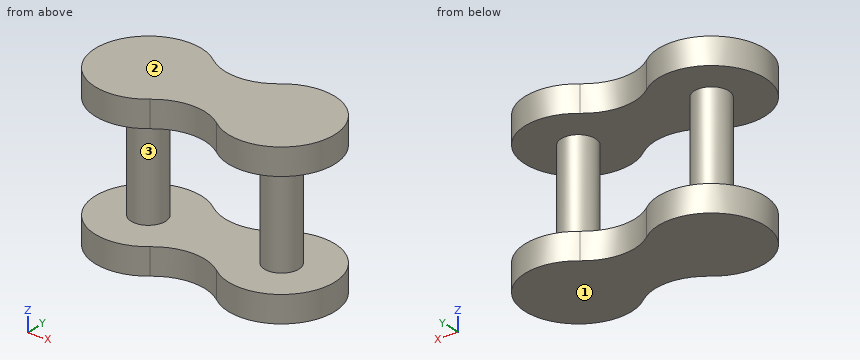
from build123d import *

# Parameters (mm, degrees)
SKETCH1_R             = 0.8255
BOSS_EXTRUDE1_DEPTH   = 2.54
BOSS_EXTRUDE1_2_DEPTH = 2.54
BOSS_EXTRUDE2_DEPTH   = 1.27


with BuildPart() as part:
    # Sketch1 → Boss-Extrude1 (new, symmetric)
    with BuildSketch(Plane.XY):
        with Locations((3.175, 0)):
            Circle(SKETCH1_R)
    extrude(amount=BOSS_EXTRUDE1_DEPTH, both=True)



with BuildPart() as body_2:
    # Sketch1 → Boss-Extrude1 2 (new, symmetric)
    with BuildSketch(Plane.XY):
        with Locations((-3.175, 0)):
            Circle(SKETCH1_R)
    extrude(amount=BOSS_EXTRUDE1_2_DEPTH, both=True)


with BuildPart() as part_1:
    add(part.part)

    add(body_2.part)  # Boss-Extrude2 merges body 2
    # Sketch2 → Boss-Extrude2 (add)
    with BuildSketch(Plane.XY.offset(2.54)):
        with BuildLine():
            ThreePointArc((1.5875, -1.982786864), (5.715, 0), (1.5875, 1.982786864))
            ThreePointArc((1.5875, 1.982786864), (0, 1.425573729), (-1.5875, 1.982786864))
            ThreePointArc((-1.5875, 1.982786864), (-5.715, 0), (-1.5875, -1.982786864))
            ThreePointArc((-1.5875, -1.982786864), (0, -1.425573729), (1.5875, -1.982786864))
        make_face()
    boss_extrude2 = extrude(amount=BOSS_EXTRUDE2_DEPTH)

    # Mirror1: Boss-Extrude2 across plane
    add(boss_extrude2.mirror(Plane.XY))


solid = part_1.part
Read the model definition and answer for the solid it produces. Units are mm, in the model's axes. Face numbers are marked on the shaded views. Coordinates: 2 decimals unless noted, no trailing zeros. Loops run counter-clockwise (first coordinate to the right, second up) from the corner with the lowest first, then second, coordinate; pieces in that order, holes last.
Q1. Consider probe 1 along Z at (x, y) = (-2.75, -1.7); probe 2 along X at (y, z) = (-0.7, -1.5); probe 3 along X at (y, z) = (0.45, 3). Determine where each line is inside the solid, lowest interval first.
Q2. The part is cut by section D-D on z = -0.25. Write down the section's boundary in (x, y) (1 decimal), and give its area (3 significant figures).
Q3. The part is cut by section A-A on y = 0. Write down the section's boundary in (x, z) (1 decimal).
Q4. The part is cut by section C-C on y = -2.2. Write down the section's boundary in (x, z), and give its area (3 significant figures).
Q5. The mould has two halves that part along Z. Classify the marked faces 1, 2 and 3: +Z half, -Z half, draft (parallel to the pull), parting line (faces both ways), or undercut.
Q6. The part is cut by section B-B on x = 1.75. Write down the section's boundary in (y, z).
Results below:
1. probe 1: z = -3.81 to -2.54, 2.54 to 3.81
1. probe 2: x = -3.61 to -2.74, 2.74 to 3.61
1. probe 3: x = -5.67 to 5.67
2. outline: circle Ø1.7 at (-3.2, 0); circle Ø1.7 at (3.2, 0)
2. area: 4.28 mm2
3. outline: (-5.7, -3.8) - (5.7, -3.8) - (5.7, -2.5) - (4, -2.5) - (4, 2.5) - (5.7, 2.5) - (5.7, 3.8) - (-5.7, 3.8) - (-5.7, 2.5) - (-4, 2.5) - (-4, -2.5) - (-5.7, -2.5) - close; hole (-2.3, -2.5) - (2.3, -2.5) - (2.3, 2.5) - (-2.3, 2.5) - close
4. outline: (-4.44, -3.81) - (-1.91, -3.81) - (-1.91, -2.54) - (-4.44, -2.54) - close; (-4.44, 2.54) - (-1.91, 2.54) - (-1.91, 3.81) - (-4.44, 3.81) - close; (1.91, -3.81) - (4.44, -3.81) - (4.44, -2.54) - (1.91, -2.54) - close; (1.91, 2.54) - (4.44, 2.54) - (4.44, 3.81) - (1.91, 3.81) - close
4. area: 12.9 mm2
5. face 1: -Z half
5. face 2: +Z half
5. face 3: undercut
6. outline: (-2.1, -3.81) - (2.1, -3.81) - (2.1, -2.54) - (-2.1, -2.54) - close; (-2.1, 2.54) - (2.1, 2.54) - (2.1, 3.81) - (-2.1, 3.81) - close
